Build history of the part. All positions in model axes, mm. Face numbers are marked on the shaded views. A direction names the side the tool comes from. Coordinates: 2 decimals unless noted, no trailing zeros. Order: outer loops, then holes, each group sorted by start corner. A loop starts at its lowest first (then second) coordinate and runs counter-clockwise, first axis right, second up. Notation, with made-up numbers: (30, -15) -> (74, -15) arc R19 cw to (74, -10) -> close; hole circle Ø7 at (69, 8.25). An arc over 180 degrees is marked (long way). Write each question's results on one line, items separated by ' | '.
from build123d import *

# Parameters (mm, degrees)
F0_W      = 50.8
F0_H      = 88.9000027377
F1_DEPTH  = 69.85
F2_R      = 20.0980289244
F3_DEPTH  = 6.35
F4_R      = 17.4104320073
F5_DEPTH  = 6.35
F6_W      = 4.6012029052
F6_H      = 5.6705921888
F6_W_2    = 4.0045529604
F6_H_2    = 3.7587732077
F7_DEPTH  = 8.89
F8_W      = 27.7972370386
F8_H      = 54.1314678267
F8_W_2    = 25.7490221411
F8_H_2    = 53.8388649002
F8_W_3    = 24.8712147586
F8_H_3    = 53.5462619737
F9_DEPTH  = 3.81
F10_W     = 27.7972389013
F10_H     = 54.7166722827
F10_W_2   = 26.0416157544
F10_H_2   = 54.4240698218
F11_DEPTH = 3.81
F12_W     = 3.2980442047
F12_H     = 45.0437162071
F12_W_2   = 2.8579700738
F12_H_2   = 45.5747190863
F12_W_3   = 2.8833756223
F12_H_3   = 44.0509710461
F13_DEPTH = 5.08
F14_W     = 2.9260246083
F14_H     = 43.5977773741
F14_W_2   = 3.8038305938
F14_H_2   = 42.7199658006
F15_DEPTH = 5.08


with BuildPart() as f1:
    # F0 (on Top) → F1 (new body)
    with BuildSketch(Plane.XY):
        Polygon((87.2851201832, 80.4412277794), (-90.5148798168, 80.4412277794), (-90.5148798168, 29.6412277794), (36.4851201832, 29.6412277794), (87.2851201832, 29.6412277794), align=None)
        with Locations((61.8851201832, -14.8087735895)):
            Rectangle(F0_W, F0_H)
    extrude(amount=F1_DEPTH)

    # F2 (on Top) → F3 (cut)
    with BuildSketch(Plane.XY):
        with Locations((-17.8680513054, 57.9398013651)):
            Circle(F2_R)
    extrude(amount=F3_DEPTH, mode=Mode.SUBTRACT)

    # F4 (on face) → F5 (cut)
    with BuildSketch(Plane.XY.offset(69.85)):
        with Locations((-32.23175928, 57.2901628911)):
            Circle(F4_R)
    extrude(amount=-F5_DEPTH, mode=Mode.SUBTRACT)

    # F6 (on face) → F7 (join)
    with BuildSketch(Plane.XY.offset(69.85)):
        with Locations((-49.2636710405, 74.4159296155)):
            Rectangle(F6_W, F6_H)
        with Locations((-18.4165723622, 75.5769610405)):
            Rectangle(F6_W_2, F6_H_2)
    extrude(amount=F7_DEPTH)

    # F8 (on face) → F9 (join)
    with BuildSketch(Plane.XZ.offset(-29.6412277794)):
        with Locations((-65.6948313117, 35.5044952594)):
            Rectangle(F8_W, F8_H)
        with Locations((-28.3880112693, 35.3581937961)):
            Rectangle(F8_W_2, F8_H_2)
        with Locations((7.7484010253, 35.2118923329)):
            Rectangle(F8_W_3, F8_H_3)
    extrude(amount=F9_DEPTH)

    # F10 (on face) → F11 (join)
    with BuildSketch(Plane(origin=(36.4851201832, 0, 0), x_dir=(0, -1, 0), z_dir=(-1, 0, 0))):
        with Locations((-0.9502042085, 34.9192901049)):
            Rectangle(F10_W, F10_H)
        with Locations((38.8437379152, 35.0655913353)):
            Rectangle(F10_W_2, F10_H_2)
    extrude(amount=F11_DEPTH)

    # F12 (on face) → F13 (join)
    with BuildSketch(Plane.XZ.offset(-29.6412277794)):
        with Locations((-56.999836117, 35.8716500923)):
            Rectangle(F12_W, F12_H)
        with Locations((-20.7188213244, 36.1371515319)):
            Rectangle(F12_W_2, F12_H_2)
        with Locations((14.2113375477, 35.3752775118)):
            Rectangle(F12_W_3, F12_H_3)
    extrude(amount=F13_DEPTH)

    # F14 (on face) → F15 (join)
    with BuildSketch(Plane(origin=(36.4851201832, 0, 0), x_dir=(0, -1, 0), z_dir=(-1, 0, 0))):
        with Locations((7.9741724767, 35.7970981859)):
            Rectangle(F14_W, F14_H)
        with Locations((46.7440057546, 35.6507943943)):
            Rectangle(F14_W_2, F14_H_2)
    extrude(amount=F15_DEPTH)


solid = f1.part
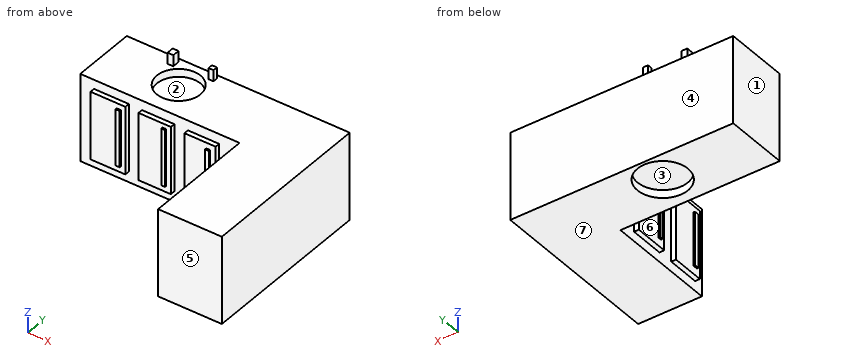
Item 1: Slice it at D-D, the plane x = 40. List the corners of the cut face in (y, z).
Answer:
outline: (-59.26, 0) -> (80.44, 0) -> (80.44, 69.85) -> (-59.26, 69.85) -> close
Item 2: Pull direction Y, two halves, no side cores. Call the marked faces 4, 5, 6 and 7: released by +Y, released by -Y, zero draft, split by the parting line, or undercut.
Answer:
face 4: released by +Y | face 5: released by -Y | face 6: undercut | face 7: zero draft
Item 3: Tool access for the marked faces 1, 2 and 3: list every direction of +Z, -Z, +X, -X, +Y, -Y with a clear straight run to the whole face (end or side of a thin tool).
Answer:
face 1: +Z, -Z, -X, +Y, -Y | face 2: +Z | face 3: -Z
Item 4: Slice it at B-B, the plane y = 5. List the corners of the cut face in (x, z), and give its area (3 significant figures).
Answer:
outline: (32.68, 7.56) -> (36.49, 7.56) -> (36.49, 0) -> (87.29, 0) -> (87.29, 69.85) -> (36.49, 69.85) -> (36.49, 62.28) -> (32.68, 62.28) -> close | area: 3,760 mm^2
Item 5: Slice it at A-A, the plane x = -63.5. List the corners of the cut face in (y, z).
Answer:
outline: (25.83, 8.44) -> (29.64, 8.44) -> (29.64, 0) -> (80.44, 0) -> (80.44, 69.85) -> (29.64, 69.85) -> (29.64, 62.57) -> (25.83, 62.57) -> close
Item 6: Drill centre lines: line 1 (Y direction, x = 35, z = 41); line 2 (Z direction, x = 16, y = 62); line 3 (Y direction, x = -83, z = 69). Where is each one in solid material? Low to high. Write a range as from..to.
Answer:
line 1: y = -51.86..-25.82, -12.95..14.85, 29.64..80.44 | line 2: z = 0..69.85 | line 3: y = 29.64..80.44
Item 7: Pin check, flat tips, straight feed: pin 1 (10 mm diameter, centred on x = -33.5, z = 17.5, fed in from -Y); pin 2 (1.1 mm diameter, centred on y = 27, z = 45.5, fed in from -X); pin 3 (1 mm diameter, centred on y = -20.5, z = 63.5, fed in from -X). Stop position of each tip, or through.
Answer:
pin 1: stops at y = 25.83 | pin 2: stops at x = -79.59 | pin 3: stops at x = 36.49
Item 8: Slice it at C-C, the plane z = 67.5. List the corners of the cut face in (x, y), and give its area (3 significant figures).
Answer:
outline: (-90.51, 29.64) -> (36.49, 29.64) -> (36.49, -59.26) -> (87.29, -59.26) -> (87.29, 80.44) -> (-90.51, 80.44) -> close; hole circle Ø34.82 at (-32.23, 57.29) | area: 12,600 mm^2
